Check sheet for the modelled part. Datum: model origin and axes. Units: mm. Face numbers are marked on the shaded views. A direction names the side the tool comes from. Round coordinates to 2 decimals unless told otherwise and drop trailing zeros. Order: outer loops, then holes, each group sorted by start corner. A loop starts at its lowest first (then second) coordinate and runs counter-clockwise, first axis right, second up. Notation, with made-up numbers: (86, 33.5) -> (132, 33.5) arc R22 cw to (132, 52.5) -> close; hole circle Ø8 at (-38.5, 49.5). An arc over 180 degrees is marked (long way). Answer in a Markdown table with one row per item.
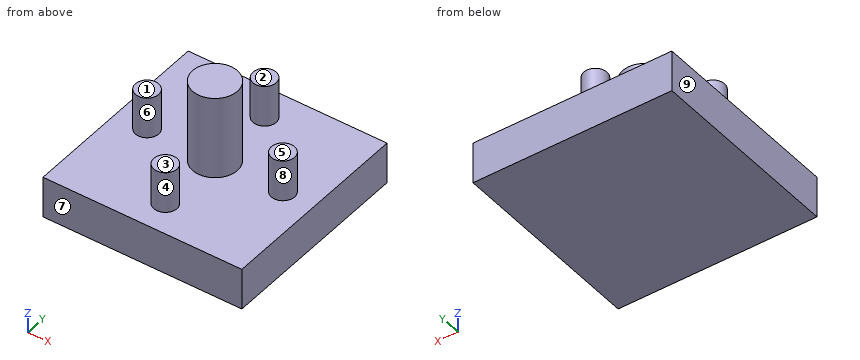
```python
from build123d import *

# Parameters (mm, degrees)
F0_W     = 120
F0_H     = 120
F1_DEPTH = 25
F2_R     = 7
F3_DEPTH = 25
F4_R     = 13.5
F5_DEPTH = 50


with BuildPart() as f1:
    # F0 (on Top) → F1 (new body)
    with BuildSketch(Plane.XY):
        Rectangle(F0_W, F0_H)
    extrude(amount=F1_DEPTH)

    # F2 (on face) → F3 (join)
    with BuildSketch(Plane.XY.offset(25)):
        with Locations((0, 41)):
            Circle(F2_R)
        with Locations((-41, 0)):
            Circle(F2_R)
        with Locations((0, -41)):
            Circle(F2_R)
        with Locations((41, 0)):
            Circle(F2_R)
    extrude(amount=F3_DEPTH)

    # F4 (on face) → F5 (join)
    with BuildSketch(Plane.XY.offset(25)):
        Circle(F4_R)
    extrude(amount=F5_DEPTH)


solid = f1.part
```
(1) Depth check by flat-ended pin: pin 1 Ø10 at (x, z) = (4, 37) entering from -Y; pin 2 Ø4 at (x, y) = (40.5, 0) entering from +Z; pin 3 Ø1 at (y, z) = (-45.5, 43.5) entering from -X. Enter the tip coordinate at first touch or a pass-through.
Solutions:
| item | result |
|---|---|
| pin 1 | y = -48 |
| pin 2 | z = 50 |
| pin 3 | x = -5.74 |
(2) Tool access check on the marked faces 1, 2, 3, 4 and 5. Record the directions out of +Z, -Z, +X, -X, +Y, -Y that give a thin tool (end or side, any length) a straight path to the whole face; none if there is none.
Solutions:
| item | result |
|---|---|
| face 1 | +Z, -X, +Y, -Y |
| face 2 | +Z, +X, -X, +Y |
| face 3 | +Z, +X, -X, -Y |
| face 4 | +Z |
| face 5 | +Z, +X, +Y, -Y |
(3) Scan lines: probe 1 along Z at (x, y) = (-20, -49); probe 2 along X at (y, z) = (-5.5, 39); probe 3 along X at (y, z) = (6, 35). Record each from-to range of solid material in increasing order. Write a range as from..to.
Solutions:
| item | result |
|---|---|
| probe 1 | 0..25 |
| probe 2 | -45.33..-36.67, -12.33..12.33, 36.67..45.33 |
| probe 3 | -44.61..-37.39, -12.09..12.09, 37.39..44.61 |
(4) Section check B-B on x = -41. Record the boundary of the cut face in (y, z).
Solutions:
| item | result |
|---|---|
| outline | (-60, 0) -> (60, 0) -> (60, 25) -> (7, 25) -> (7, 50) -> (-7, 50) -> (-7, 25) -> (-60, 25) -> close |
(5) Section check A-A on y = 0. Record the boundary of the cut face in (x, z).
Solutions:
| item | result |
|---|---|
| outline | (-60, 0) -> (60, 0) -> (60, 25) -> (48, 25) -> (48, 50) -> (34, 50) -> (34, 25) -> (13.5, 25) -> (13.5, 75) -> (-13.5, 75) -> (-13.5, 25) -> (-34, 25) -> (-34, 50) -> (-48, 50) -> (-48, 25) -> (-60, 25) -> close |
(6) Draft check along X on the marked faces 6, 7, 8 and 9. Enter one of: pulls with the +X half, pulls with the -X half, needs draft (parallel to the pull), parting line crosses it, or undercut.
Solutions:
| item | result |
|---|---|
| face 6 | undercut |
| face 7 | needs draft |
| face 8 | undercut |
| face 9 | pulls with the -X half |
(7) Section check C-C on z = 32. Record the boundary of the cut face in (x, y), plus the area to 3 significant figures.
Solutions:
| item | result |
|---|---|
| outline | circle Ø14 at (-41, 0); circle Ø27 at (0, 0); circle Ø14 at (0, -41); circle Ø14 at (0, 41); circle Ø14 at (41, 0) |
| area | 1,190 mm^2 |
